from build123d import *

# Parameters (mm, degrees)
F3_SIZE = 4.99999
F4_R    = 5


# Not quite as in the source:
# - a fillet or chamfer is up to 0.001 mm smaller than in the source, because OpenCascade refuses the exact size


with BuildPart() as f1:
    # F0 (on Front) → F1 (revolve)
    with BuildSketch(Plane.XZ):
        with BuildLine():
            Line((0, 11.4077670069), (0, 0))
            Line((0, 0), (75, 0))
            Line((75, 0), (75, 15))
            Line((75, 15), (50, 15))
            Line((50, 15), (50, 30))
            Line((50, 30), (40, 30))
            Line((40, 30), (40, 16.4077670069))
            ThreePointArc((40, 16.4077670069), (38.5355339059, 12.872233101), (35, 11.4077670069))
            Line((35, 11.4077670069), (0, 11.4077670069))
        make_face()
    revolve(axis=Axis((37.5, 0, 0), (-1, 0, 0)))

    # F2: F1 across face


with BuildPart() as f1_1:
    add(f1.part)
    add(f1.part.mirror(Plane(origin=(0, 0, 0), x_dir=(0, -1, 0), z_dir=(-1, 0, 0))))

    # F3 (size 5 in the source; OpenCascade refuses exactly that, so slightly less here)
    f3_edges = [f1_1.edges().sort_by_distance(p)[0] for p in [
        (-40, 0, -30),
        (-75, 0, -15),
        (-50, 0, -30),
        (40, 0, -30),
        (40, 0, -16.407767),
        (-35, 0, -11.407767),
        (35, 0, -11.407767),
        (75, 0, -15),
        (50, 0, -30),
        (-40, 0, -16.407767),
        (-50, 0, -15),
        (50, 0, -15),
    ]]
    chamfer(f3_edges, length=F3_SIZE)

    # F4
    f4_edges = [f1_1.edges().sort_by_distance(p)[0] for p in [
        (-75, 0, -10.00001),
        (75, 0, -10.00001),
    ]]
    fillet(f4_edges, radius=F4_R)


solid = f1_1.part
The listing builds one solid part. Answer for the finished solid, in the listing's coordinates (mm). A direction names the side the tool comes from. Coordinates: 2 decimals unless noted, no trailing zeros. Loops run counter-clockwise (first coordinate to the right, second up) from the corner with the lowest first, then second, coordinate; pieces in that order, holes last. Notation, with made-up numbers: M -5,25 L 7,25 A12 ccw 7,33 Z; hole C -15,45 d9. An arc over 180 degrees is marked long. Answer in a Markdown table with one row per item.
1) Determine the mould class of faces 4 (the conical face through (-49.69, 7.6, 24.14)), 5 (the conical face through (-40.243, 7.582, 24.077)), 6 (the conical face through (73.364, -11.359, -2.522)), 7 (the conical face through (40.31, 7.6, 24.14)) for opening direction X: released by +X, released by -X, zero draft, split by the parting line, or undercut.
Answers below:
| item | result |
|---|---|
| face 4 | released by -X |
| face 5 | undercut |
| face 6 | released by +X |
| face 7 | undercut |
2) Find section B-B (x = 37). Determine the outline of the cut face in (y, z).
Answers below:
| item | result |
|---|---|
| outline | C 0,0 d23.65 |
3) Which of the six approach directions +Z, -Z, +X, -X, +Y, -Y give full straight-line access (tool end or side, diameter ignored) to faces 1 (the cylindrical face through (62.395, 0.66, -14.985)), 2 (the cylindrical face through (-62.395, 0.66, -14.985)), 3 (the flat face through (-40, -5, 16))?
Answers below:
| item | result |
|---|---|
| face 1 | +X |
| face 2 | -X |
| face 3 | none |
4) Given pin 1 (10 mm diameter, centred on x = 51.5, y = 0.5, fed in from +Z); pin 2 (1 mm diameter, centred on x = -32.5, z = -7, fed in from +Y); pin 3 (1.5 mm diameter, centred on y = 21, z = 18, fed in from +X), each flat-ended and moving along its own axis, determine where each tip first touches the part or whether it passes through.
Answers below:
| item | result |
|---|---|
| pin 1 | z = 28.5 |
| pin 2 | y = 9.37 |
| pin 3 | x = 48.09 |
5) Find section A-A (x = 2). Determine the outline of the cut face in (y, z).
Answers below:
| item | result |
|---|---|
| outline | C 0,0 d22.82 |
6) Find the intervals of material crossed by probe 1 along X at (y, z) = (24, -3.5); probe 2 along Y at (x, z) = (49.5, 5) (3 decimals); probe 3 along X at (y, z) = (-18.5, 19.5), in increasing order.
Answers below:
| item | result |
|---|---|
| probe 1 | -50 to -40, 40 to 50 |
| probe 2 | -25.005 to 25.005 |
| probe 3 | -48.12 to -41.88, 41.88 to 48.12 |
